```python
from build123d import *

# Parameters (mm, degrees)
BOSS_EXTRUDE1_DEPTH = 12
SKETCH2_W           = 5.5
SKETCH2_H           = 13
SKETCH2_W_2         = 1
SKETCH2_H_2         = 11.5
CUT_EXTRUDE1_DEPTH  = 10
SKETCH3_W           = 15.4
SKETCH3_H           = 7.5
SKETCH3_W_2         = 12.9
SKETCH3_H_2         = 1
CUT_EXTRUDE2_DEPTH  = 10
SKETCH4_R           = 5
BOSS_EXTRUDE2_DEPTH = 12
BOSS_EXTRUDE2_TAPER = 3


with BuildPart() as part:
    # Sketch1 → Boss-Extrude1 (new, symmetric)
    with BuildSketch(Plane(origin=(0, 0, 0), x_dir=(1, 0, 0), z_dir=(0, 1, 0))):
        with BuildLine():
            Line((-48, -16.5), (48, -16.5))
            ThreePointArc((48, -16.5), (51.535533906, -15.035533906), (53, -11.5))
            Line((53, -11.5), (53, 11.5))
            ThreePointArc((53, 11.5), (51.535533906, 15.035533906), (48, 16.5))
            Line((48, 16.5), (-48, 16.5))
            ThreePointArc((-48, 16.5), (-51.535533906, 15.035533906), (-53, 11.5))
            Line((-53, 11.5), (-53, -11.5))
            ThreePointArc((-53, -11.5), (-51.535533906, -15.035533906), (-48, -16.5))
        make_face()
    extrude(amount=BOSS_EXTRUDE1_DEPTH, both=True)

    # Sketch2 → Cut-Extrude1 (cut)
    # profile 1 of 3: a face of its own
    with BuildSketch(Plane(origin=(0, 12, 0), x_dir=(1, 0, 0), z_dir=(0, 1, 0))):
        with Locations((15.25, 0)):
            Rectangle(SKETCH2_W, SKETCH2_H)
        with Locations((16.75, 0)):
            Rectangle(SKETCH2_W_2, SKETCH2_H_2, mode=Mode.SUBTRACT)
    # profile 2 of 3: a face of its own
    with BuildSketch(Plane(origin=(0, 12, 0), x_dir=(1, 0, 0), z_dir=(0, 1, 0))):
        with Locations((-8.25, 0)):
            Rectangle(SKETCH2_W, SKETCH2_H)
        with Locations((-6.75, 0)):
            Rectangle(SKETCH2_W_2, SKETCH2_H_2, mode=Mode.SUBTRACT)
    # profile 3 of 3: a face of its own
    with BuildSketch(Plane(origin=(0, 12, 0), x_dir=(1, 0, 0), z_dir=(0, 1, 0))):
        with Locations((-31.75, 0)):
            Rectangle(SKETCH2_W, SKETCH2_H)
        with Locations((-30.25, 0)):
            Rectangle(SKETCH2_W_2, SKETCH2_H_2, mode=Mode.SUBTRACT)
    extrude(amount=-CUT_EXTRUDE1_DEPTH, mode=Mode.SUBTRACT)

    # Sketch3 → Cut-Extrude2 (cut)
    with BuildSketch(Plane.ZY.offset(53)):
        Rectangle(SKETCH3_W, SKETCH3_H)
        with Locations((0, 2)):
            Rectangle(SKETCH3_W_2, SKETCH3_H_2, mode=Mode.SUBTRACT)
    extrude(amount=-CUT_EXTRUDE2_DEPTH, mode=Mode.SUBTRACT)

    # Sketch4 → Boss-Extrude2 (add)
    with BuildSketch(Plane(origin=(53, 0, 0), x_dir=(0, 0, -1), z_dir=(1, 0, 0))):
        Circle(SKETCH4_R)
    extrude(amount=BOSS_EXTRUDE2_DEPTH, taper=BOSS_EXTRUDE2_TAPER)


solid = part.part
```
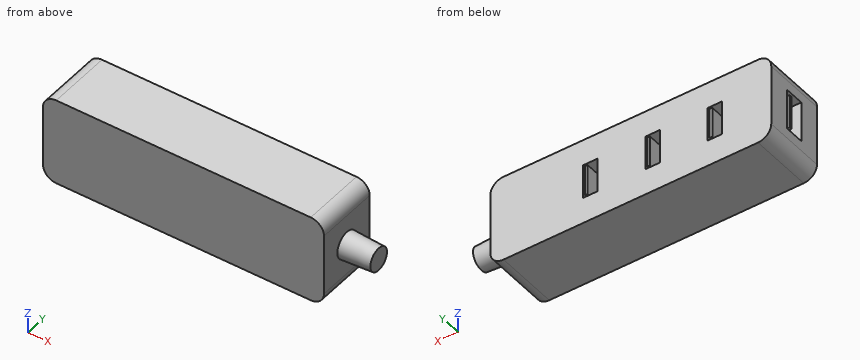
Verification items for the finished model (mm, model axes). Give positions to 0.01 mm unless a question says otherwise; leave off trailing zeros. Order: outer loops, then holes, each group sorted by start corner. A loop starts at its lowest first (then second) coordinate and runs counter-clockwise, first axis right, second up. Notation, with made-up numbers: (-38.5, 33) - (-25.5, 33) arc R15 cw to (-25.5, 59) - close; hole circle Ø2 at (26.25, 12.25). An arc over 180 degrees is marked (long way). Answer as CSV lines item,"result". Start each with the question number.
Item 1: Gauge pin test, flat ends, axial feed: pin 1 (1.6 mm diameter, centred on x = 14, z = 0.5, fed in from +Y); pin 2 (1 mm diameter, centred on y = -4, z = -11.5, fed in from +X). Record the tip position at first contact, or that the pin passes through.
Item 2: Section check C-C, the plane z = -10. Record the boundary of the cut face in (x, y), plus the area to 3 significant figures.
Item 3: Material ranges on L1, parallel to Z at x = -30, y = 7.25; L2, parallel to Z at x = 16, y = 8.25; L3, parallel to X at y = 1, z = -12, recorded low to high.
Item 4: Section check A-A, the plane y = 8.75. State how many separate pieces and enclosed holes the cut face has, plus the area to 3 significant figures.
Item 5: Section check B-B, the plane y = -10.25. Record the boundary of the cut face in (x, z).
Filled in:
1,pin 1,"y = 2"
1,pin 2,"x = 53"
2,outline,"(-53, -12) - (53, -12) - (53, 12) - (-53, 12) - close"
2,area,"2,540 mm^2"
3,L1,"-16.5 to -6.5, -5.75 to 5.75, 6.5 to 16.5"
3,L2,"-16.5 to -6.5, 6.5 to 16.5"
3,L3,"-52.97 to 52.97"
4,separate pieces,"4"
4,enclosed holes,"3"
4,area,"3,300 mm^2"
5,outline,"(-53, -11.5) arc R5 ccw to (-48, -16.5) - (48, -16.5) arc R5 ccw to (53, -11.5) - (53, 11.5) arc R5 ccw to (48, 16.5) - (-48, 16.5) arc R5 ccw to (-53, 11.5) - close"
